Part model, mm, in its own coordinate system. A direction names the side the tool comes from. Coordinates: 2 decimals unless noted, no trailing zeros. Loops run counter-clockwise (first coordinate to the right, second up) from the corner with the lowest first, then second, coordinate; pieces in that order, holes last. Notation, with made-up numbers: M 7.5,43 L 49.5,43 A23 ccw 49.5,60 Z; hole C 67.25,11.5 d9. An arc over 180 degrees is marked long. Answer as a JSON object with one key per item and string values. Group by question number.
1. Mould opens along X. For faces 1 (the face through (-22.4, 28, 50)), 2 (the face through (-57.35, 51.39, -38.51)), 3 (the face through (-25, 42, -1)), 4 (the face through (-22, 41, 1)) say: released by +X, released by -X, zero draft, split by the parting line, or undercut.
2. Saw through at B-B on z = 16. Write the cut outline in (x, y).
3. Drop flat-ended pins along their axis: pin 1 Ø6 at (y, z) = (35.5, -25) entering from -X; pin 2 Ø1 at (x, z) = (-38, -38) entering from -Y; pin 3 Ø1.5 at (x, y) = (-78.97, 38.65) entering from -Z; pin 4 Ø10 at (x, z) = (-44.5, -30.5) entering from +Y. Give the stop position or say it passes through.
4. 3-axis set-ups, long thin cutter, end or side, ignore diameter. For faces 5 (the face through (-52, 48, -37.5)), 6 (the face through (-56.574, 38.891, 7.014)), 7 (the face through (-52, 41, 8)), 8 (the face through (1, 2, -1)): which of +Z, -Z, +X, -X, +Y, -Y reach the whole face in a straight line?
5. Saw through at A-A on y = 58. Write the cut outline in (x, z).
6. Drill centre lines: L1, parallel to Y at x = -61.65, z = 7.1; L2, parallel to Z at x = -44.5, y = 57.5; L3, parallel to X at y = 38.65, z = 7.1. Where is each one in solid material? Low to high.
7. Saw through at C-C on y = 7. Write the cut outline in (x, z), then the cut area to 3 significant figures.
from build123d import *

# Parameters (mm, degrees)
SKETCH_1_W                   = 50
SKETCH_1_H                   = 100
EXTRUDE_1_DEPTH              = 2
SKETCH_2_W                   = 3
SKETCH_2_H                   = 100
EXTRUDE_2_DEPTH              = 80
SKETCH_3_W                   = 2
SKETCH_3_H                   = 66.7
EXTRUDE_3_DEPTH              = 70
CUT_EXTRUDE_4_REACH          = 162.465
SKETCH_8_W                   = 2
SKETCH_8_H                   = 66.7
EXTRUDE_4_DEPTH              = 70
CUT_EXTRUDE_5_REACH          = 140.25
HOLE_WIZARD_M3_1_D           = 2.5
HOLE_WIZARD_M3_1_DEPTH       = 2
HOLE_WIZARD_M3_1_CSINK_D     = 3.05
HOLE_WIZARD_M3_1_CSINK_ANGLE = 90
FILLET_1_R                   = 2
CUT_EXTRUDE_6_REACH          = 140.25
SKETCH_12_R                  = 11
CUT_EXTRUDE_7_REACH          = 162.465
SKETCH_13_R                  = 14.5
SKETCH_14_W                  = 2
SKETCH_14_H                  = 66.7
EXTRUDE_5_DEPTH              = 70
CUT_EXTRUDE_8_REACH          = 156.14
SKETCH_15_R                  = 5.1
CUT_EXTRUDE_9_DEPTH          = 155.140358116
CUT_EXTRUDE_9_DEPTH_BACK     = 155.140358116
SKETCH_19_W                  = 2
SKETCH_19_H                  = 66.7
CUT_EXTRUDE_10_DEPTH         = 119.844436134
FILLET_2_R                   = 2


with BuildPart() as part:
    # 草图1 → 凸台-拉伸1 (new body)
    with BuildSketch(Plane(origin=(0, 0, 0), x_dir=(1, 0, 0), z_dir=(0, 1, 0))):
        Rectangle(SKETCH_1_W, SKETCH_1_H)
    extrude(amount=EXTRUDE_1_DEPTH)

    # 草图2 → 凸台-拉伸2 (add)
    with BuildSketch(Plane(origin=(0, 2, 0), x_dir=(1, 0, 0), z_dir=(0, 1, 0))):
        with Locations((-23.5, 0)):
            Rectangle(SKETCH_2_W, SKETCH_2_H)
    extrude(amount=EXTRUDE_2_DEPTH)

    # 草图3 → 凸台-拉伸3 (add)
    with BuildSketch(Plane.ZY.offset(25)):
        with Locations((-49, 48.65)):
            Rectangle(SKETCH_3_W, SKETCH_3_H)
    extrude(amount=EXTRUDE_3_DEPTH)

    # 草图4 → 切除-拉伸4 (cut, up to next)
    with BuildSketch(Plane(origin=(0, 0, -50), x_dir=(-1, 0, 0), z_dir=(0, 0, -1)), mode=Mode.PRIVATE) as cut_extrude_4_sk1:
        with BuildLine():
            Line((95, 82), (61.65, 82))
            ThreePointArc((61.65, 82), (85.232011153, 72.232011153), (95, 48.65))
            Line((95, 48.65), (95, 82))
        make_face()
    cut_extrude_4_tool1 = extrude(cut_extrude_4_sk1.sketch, amount=-CUT_EXTRUDE_4_REACH, mode=Mode.PRIVATE) & part.part
    # 草图4 → 切除-拉伸4 (cut, up to next)
    with BuildSketch(Plane(origin=(0, 0, -50), x_dir=(-1, 0, 0), z_dir=(0, 0, -1)), mode=Mode.PRIVATE) as cut_extrude_4_sk2:
        with BuildLine():
            ThreePointArc((95, 48.65), (85.232011153, 25.067988847), (61.65, 15.3))
            Line((61.65, 15.3), (95, 15.3))
            Line((95, 15.3), (95, 48.65))
        make_face()
    cut_extrude_4_tool2 = extrude(cut_extrude_4_sk2.sketch, amount=-CUT_EXTRUDE_4_REACH, mode=Mode.PRIVATE) & part.part
    add(cut_extrude_4_tool1.solids().sort_by_distance((-87.550679, 74.550679, -50))[0], mode=Mode.SUBTRACT)
    add(cut_extrude_4_tool2.solids().sort_by_distance((-87.550679, 22.749321, -50))[0], mode=Mode.SUBTRACT)

    # 草图8 → 凸台-拉伸4 (add)
    with BuildSketch(Plane.ZY.offset(25)):
        with Locations((7, 48.65)):
            Rectangle(SKETCH_8_W, SKETCH_8_H)
    extrude(amount=EXTRUDE_4_DEPTH)

    # 草图9 → 切除-拉伸5 (cut, up to next)
    with BuildSketch(Plane.XY.offset(8), mode=Mode.PRIVATE) as cut_extrude_5_sk1:
        with BuildLine():
            ThreePointArc((-95, 48.65), (-85.232011153, 72.232011153), (-61.65, 82))
            Line((-61.65, 82), (-95, 82))
            Line((-95, 82), (-95, 48.65))
        make_face()
    cut_extrude_5_tool1 = extrude(cut_extrude_5_sk1.sketch, amount=-CUT_EXTRUDE_5_REACH, mode=Mode.PRIVATE) & part.part
    # 草图9 → 切除-拉伸5 (cut, up to next)
    with BuildSketch(Plane.XY.offset(8), mode=Mode.PRIVATE) as cut_extrude_5_sk2:
        with BuildLine():
            ThreePointArc((-61.65, 15.3), (-85.232011153, 25.067988847), (-95, 48.65))
            Line((-95, 48.65), (-95, 15.3))
            Line((-95, 15.3), (-61.65, 15.3))
        make_face()
    cut_extrude_5_tool2 = extrude(cut_extrude_5_sk2.sketch, amount=-CUT_EXTRUDE_5_REACH, mode=Mode.PRIVATE) & part.part
    add(cut_extrude_5_tool1.solids().sort_by_distance((-87.550679, 74.550679, 8))[0], mode=Mode.SUBTRACT)
    add(cut_extrude_5_tool2.solids().sort_by_distance((-87.550679, 22.749321, 8))[0], mode=Mode.SUBTRACT)

    # M3 螺纹孔1
    with Locations(Plane.XY.offset(8)):
        with Locations((-78.970508076, 38.65), (-61.65, 68.65), (-44.329491924, 38.65)):
            CounterSinkHole(HOLE_WIZARD_M3_1_D / 2, HOLE_WIZARD_M3_1_CSINK_D / 2, depth=HOLE_WIZARD_M3_1_DEPTH, counter_sink_angle=HOLE_WIZARD_M3_1_CSINK_ANGLE)

    # 圆角1
    fillet_1_edges = [part.edges().sort_by_distance(p)[0] for p in [
        (-23.5, 82, 50),
        (25, 1, 50),
        (25, 1, -50),
    ]]
    fillet(fillet_1_edges, radius=FILLET_1_R)

    # 草图12 → 切除-拉伸6 (cut, up to next)
    with BuildSketch(Plane.XY.offset(8), mode=Mode.PRIVATE) as cut_extrude_6_sk1:
        with Locations((-61.65, 48.65)):
            Circle(SKETCH_12_R)
    cut_extrude_6_tool1 = extrude(cut_extrude_6_sk1.sketch, amount=-CUT_EXTRUDE_6_REACH, mode=Mode.PRIVATE) & part.part
    add(cut_extrude_6_tool1.solids().sort_by_distance((-61.65, 48.65, 8))[0], mode=Mode.SUBTRACT)

    # 草图13 → 切除-拉伸7 (cut, up to next)
    with BuildSketch(Plane(origin=(0, 0, -50), x_dir=(-1, 0, 0), z_dir=(0, 0, -1)), mode=Mode.PRIVATE) as cut_extrude_7_sk1:
        with Locations((61.65, 48.65)):
            Circle(SKETCH_13_R)
    cut_extrude_7_tool1 = extrude(cut_extrude_7_sk1.sketch, amount=-CUT_EXTRUDE_7_REACH, mode=Mode.PRIVATE) & part.part
    add(cut_extrude_7_tool1.solids().sort_by_distance((-61.65, 48.65, -50))[0], mode=Mode.SUBTRACT)

    # 草图14 → 凸台-拉伸5 (add)
    with BuildSketch(Plane.ZY.offset(25)):
        with Locations((-38.5, 48.65)):
            Rectangle(SKETCH_14_W, SKETCH_14_H)
    extrude(amount=EXTRUDE_5_DEPTH)

    # 草图15 → 切除-拉伸8 (cut, up to next)
    with BuildSketch(Plane(origin=(0, 0, -39.5), x_dir=(-1, 0, 0), z_dir=(0, 0, -1)), mode=Mode.PRIVATE) as cut_extrude_8_sk1:
        with Locations(Location((61.65, 48.65, 0), (0, 0, 90))):
            Circle(SKETCH_15_R)
    cut_extrude_8_tool1 = extrude(cut_extrude_8_sk1.sketch, amount=-CUT_EXTRUDE_8_REACH, mode=Mode.PRIVATE) & part.part
    add(cut_extrude_8_tool1.solids().sort_by_distance((-61.65, 48.65, -39.5))[0], mode=Mode.SUBTRACT)

    # 草图18 → 切除-拉伸9 (cut, two sides: drawn at the far end of the back side and taken through both)
    with BuildSketch(Plane(origin=(0, 0, -39.5), x_dir=(-1, 0, 0), z_dir=(0, 0, -1)).offset(-CUT_EXTRUDE_9_DEPTH_BACK)):
        with BuildLine():
            Line((95, 15.3), (95, 48.65))
            ThreePointArc((95, 48.65), (85.232011153, 25.067988847), (61.65, 15.3))
            Line((61.65, 15.3), (95, 15.3))
        make_face()
        with BuildLine():
            Line((95, 48.65), (95, 82))
            Line((95, 82), (61.65, 82))
            ThreePointArc((61.65, 82), (85.232011153, 72.232011153), (95, 48.65))
        make_face()
    extrude(amount=CUT_EXTRUDE_9_DEPTH + CUT_EXTRUDE_9_DEPTH_BACK, mode=Mode.SUBTRACT)

    # 草图19 → 切除-拉伸10 (cut, through all)
    with BuildSketch(Plane.ZY.offset(25)):
        with Locations((-49, 48.65)):
            Rectangle(SKETCH_19_W, SKETCH_19_H)
    extrude(amount=CUT_EXTRUDE_10_DEPTH, mode=Mode.SUBTRACT)

    # 圆角2
    fillet_2_edges = [part.edges().sort_by_distance(p)[0] for p in [
        (-23.5, 82, -50),
    ]]
    fillet(fillet_2_edges, radius=FILLET_2_R)


solid = part.part
Outcome:
{
 "1": {"face 1": "zero draft", "face 2": "undercut", "face 3": "released by -X", "face 4": "released by +X"},
 "2": {"outline": "M -25,0 L 25,0 L 25,2 L -22,2 L -22,82 L -25,82 Z"},
 "3": {"pin 1": "stops at x = -25", "pin 2": "stops at y = 15.3", "pin 3": "stops at z = -39.5", "pin 4": "passes through"},
 "4": {"face 5": "-X, +Y, -Y", "face 6": "+Z", "face 7": "+Z, -X, +Y, -Y", "face 8": "+Z, -Z, +X, +Y"},
 "5": {"outline": "M -93.66,-39.5 L -25,-39.5 L -25,-50 L -22,-50 L -22,50 L -25,50 L -25,8 L -55.86,8 L -55.86,6 L -25,6 L -25,-37.5 L -93.66,-37.5 Z; M -93.66,6 L -67.44,6 L -67.44,8 L -93.66,8 Z"},
 "6": {"L1": "y = 15.3 to 37.65, 59.65 to 67.4, 69.9 to 82", "L2": "z = -39.5 to -37.5, 6 to 8", "L3": "x = -93.47 to -80.22, -77.72 to -66.23, -57.07 to -45.58, -43.08 to -22"},
 "7": {"outline": "M -25,-50 L -22,-50 L -22,50 L -25,50 Z", "area": "300 mm²"}
}
